from build123d import *

# Parameters (mm, degrees)
F0_W        = 47.8054173291
F0_H        = 43.6823405325
F1_DEPTH    = 79.23727
F2_T1_DEPTH = 403.639522146
F3_R        = 5.08
F4_W        = 28.1929401681
F4_H        = 17.383787781
F5_DEPTH    = 83.42686


# Not quite as in the source:
# - a fillet or chamfer that OpenCascade refuses, or shapes differently, is made with other operations: its cross-section is extruded or revolved along the edge and cut away or added


with BuildPart() as f1:
    # F0 (on Front) → F1 (new body)
    with BuildSketch(Plane.XZ):
        with Locations((2.172973007, 21.8411702663)):
            Rectangle(F0_W, F0_H)
    extrude(amount=F1_DEPTH)

    # F2: fillet of radius 67.9298616849 on 1 edges, made by hand

    # F2_s2 → F2_t1 (cut)
    with BuildSketch(Plane.XZ.offset(-162.201126073)):
        with BuildLine():
            ThreePointArc((-21.7297356576, 64.8804504292), (-8.4877009093, 24.5851939655), (26.0756816715, 0))
            Line((26.0756816715, 0), (-21.7297356576, 0))
            Line((-21.7297356576, 0), (-21.7297356576, 64.8804504292))
        make_face()
    extrude(amount=F2_T1_DEPTH, mode=Mode.SUBTRACT)

    # F3
    f3_edges = [f1.edges().sort_by_distance(p)[0] for p in [
        (26.075682, -39.618635, 43.682341),
        (3.869087, -79.23727, 43.682341),
        (26.075682, -79.23727, 21.84117),
        (26.075682, 0, 21.84117),
        (3.869087, 0, 43.682341),
    ]]
    fillet(f3_edges, radius=F3_R)

    # F4 (on Top) → F5 (join)
    with BuildSketch(Plane.XY):
        with Locations((3.2873195596, -42.192241177)):
            Rectangle(F4_W, F4_H)
    extrude(amount=F5_DEPTH)


solid = f1.part
CAD build for the part. Positions are in the model's coordinates, mm. A direction names the side the tool comes from. Give positions to 0.01 mm unless a question says otherwise; leave off trailing zeros. Order: outer loops, then holes, each group sorted by start corner. A loop starts at its lowest first (then second) coordinate and runs counter-clockwise, first axis right, second up. Notation, with made-up numbers: (-6, 43.25) - (30, 43.25) arc R34 cw to (30, 79.25) - close; hole circle Ø6 at (-23.5, 13). An arc over 180 degrees is marked (long way). Answer in a Markdown table with one row per item.
1. Pull direction X, two halves, no side cores. Call faces 1 (the flat face through (6, 0, 25)), 2 (the flat face through (-10.809, -42, 14)), 3 (the cylindrical face through (24.6, -1.5, 19.6)), 4 (the flat face through (17.384, -42, 2)): pulls with the +X half, pulls with the -X half, needs draft (parallel to the pull), parting line crosses it, or undercut.
Data:
| item | result |
|---|---|
| face 1 | needs draft |
| face 2 | pulls with the -X half |
| face 3 | pulls with the +X half |
| face 4 | undercut |
2. Saw through at B-B, the plane z = 9. Give the cut face in (x, y), plus the area to 3 significant figures.
Data:
| item | result |
|---|---|
| outline | (-10.81, -50.88) - (7.58, -50.88) - (7.58, -79.24) - (21, -79.24) arc R5.08 ccw to (26.08, -74.16) - (26.08, -5.08) arc R5.08 ccw to (21, 0) - (7.58, 0) - (7.58, -33.5) - (-10.81, -33.5) - close |
| area | 1,770 mm² |
3. Saw through at C-C, the plane x = -4. Give the cut face in (y, z).
Data:
| item | result |
|---|---|
| outline | (-79.24, 19.12) - (-50.88, 19.12) - (-50.88, 0) - (-33.5, 0) - (-33.5, 19.12) - (0, 19.12) - (0, 38.6) arc R5.08 ccw to (-5.08, 43.68) - (-33.5, 43.68) - (-33.5, 83.43) - (-50.88, 83.43) - (-50.88, 43.68) - (-74.16, 43.68) arc R5.08 ccw to (-79.24, 38.6) - close |
4. Saw through at A-A, the plane y = -35. Give the cut face in (x, z), plus the area to 3 significant figures.
Data:
| item | result |
|---|---|
| outline | (-18.34, 43.68) arc R67.93 ccw to (-10.81, 27.94) - (-10.81, 0) - (17.38, 0) - (17.38, 3.37) arc R67.93 ccw to (26.08, 0) - (26.08, 38.6) arc R5.08 ccw to (21, 43.68) - (17.38, 43.68) - (17.38, 83.43) - (-10.81, 83.43) - (-10.81, 43.68) - close |
| area | 2,780 mm² |
5. Saw through at D-D, the plane y = -66. Give the cut face in (x, z), plus the area to 3 significant figures.
Data:
| item | result |
|---|---|
| outline | (-18.34, 43.68) arc R67.93 ccw to (26.08, 0) - (26.08, 38.6) arc R5.08 ccw to (21, 43.68) - close |
| area | 1,280 mm² |
6. Tool access for faces 5 (the flat face through (0, -50.884, 8)), 6 (the flat face through (-10.809, -42, 63)), 7 (the flat face through (0, -33.5, 8)), 8 (the flat face through (3, -50.884, 63)): list every direction of +Z, -Z, +X, -X, +Y, -Y with a clear straight run to the whole face (end or side of a thin tool).
Data:
| item | result |
|---|---|
| face 5 | -Z, -X, -Y |
| face 6 | +Z, -X, +Y, -Y |
| face 7 | -Z, -X, +Y |
| face 8 | +Z, +X, -X, -Y |
7. Probe probe 1 along Y at (x, z) = (7.5, 49); probe 2 along X at (y, z) = (-43, 55); probe 3 along X at (y, z) = (-47, 10). List the from-to ranges inside material, lowest first. Write a range as [from, to].
Data:
| item | result |
|---|---|
| probe 1 | y = [-50.88, -33.5] |
| probe 2 | x = [-10.81, 17.38] |
| probe 3 | x = [-10.81, 26.08] |
8. Flat gauge pins, fed straight in: pin 1 (19 mm diameter, centred on y = -46, z = 18.5, fed in from -X); pin 2 (8.5 mm diameter, centred on y = -46, z = 68.5, fed in from +X); pin 3 (10 mm diameter, centred on x = 17.5, z = 75, fed in from +Y). Where does each tip first touch, or does it go through?
Data:
| item | result |
|---|---|
| pin 1 | stops at x = -10.85 |
| pin 2 | stops at x = 17.38 |
| pin 3 | stops at y = -33.5 |
